```python
from build123d import *

# Parameters (mm, degrees)
EXTRU_MINCE1_DEPTH      = 8
ESQUISSE2_R             = 1.6
ENL_V_MAT_EXTRU_1_DEPTH = 109.260681026
ESQUISSE3_R             = 2
ENL_V_MAT_EXTRU_2_DEPTH = 5.5
ESQUISSE4_R             = 1.6
ENL_V_MAT_EXTRU_3_DEPTH = 109.260681026
ESQUISSE5_R             = 2
ENL_V_MAT_EXTRU_4_DEPTH = 5.5
ESQUISSE7_R             = 1.6
ENL_V_MAT_EXTRU_5_DEPTH = 102.558480966
ESQUISSE8_R             = 2
ENL_V_MAT_EXTRU_6_DEPTH = 5.5
CONG_1_R                = 2


with BuildPart() as part:
    # Esquisse1 → Extru.-Mince1 (new body)
    with BuildSketch(Plane(origin=(0, 0, 0), x_dir=(1, 0, 0), z_dir=(0, 1, 0))):
        with BuildLine():
            Line((0, 0), (19.803847577, 0))
            ThreePointArc((19.803847577, 0), (24.303847577, -1.205771366), (27.598076211, -4.5))
            Line((27.598076211, -4.5), (59.352341017, -59.5))
            ThreePointArc((59.352341017, -59.5), (62.646569651, -62.794228634), (67.146569651, -64))
            Line((67.146569651, -64), (86.950417228, -64))
            Line((86.950417228, -64), (86.950417228, -56))
            Line((86.950417228, -56), (67.146569651, -56))
            ThreePointArc((67.146569651, -56), (66.646569651, -55.866025404), (66.280544247, -55.5))
            Line((66.280544247, -55.5), (34.526279442, -0.5))
            ThreePointArc((34.526279442, -0.5), (28.303847577, 5.722431864), (19.803847577, 8))
            Line((19.803847577, 8), (0, 8))
            Line((0, 8), (0, 0))
        make_face()
    extrude(amount=EXTRU_MINCE1_DEPTH)

    # Esquisse2 → Enlèv. mat.-Extru.1 (cut, through all)
    with BuildSketch(Plane(origin=(0, 8, 0), x_dir=(1, 0, 0), z_dir=(0, 1, 0))):
        with Locations(Location((74.950417228, -60, 0), (0, 0, 270))):
            Circle(ESQUISSE2_R)
        with Locations(Location((12, 4, 0), (0, 0, 270))):
            Circle(ESQUISSE2_R)
    extrude(amount=-ENL_V_MAT_EXTRU_1_DEPTH, mode=Mode.SUBTRACT)

    # Esquisse3 → Enlèv. mat.-Extru.2 (cut)
    with BuildSketch(Plane.XZ):
        with Locations(Location((74.950417228, 60, 0), (0, 0, 270))):
            Circle(ESQUISSE3_R)
        with Locations(Location((12, -4, 0), (0, 0, 270))):
            Circle(ESQUISSE3_R)
    extrude(amount=-ENL_V_MAT_EXTRU_2_DEPTH, mode=Mode.SUBTRACT)

    # Esquisse4 → Enlèv. mat.-Extru.3 (cut, through all)
    with BuildSketch(Plane(origin=(0, 0, 0), x_dir=(-1, 0, 0), z_dir=(0, 0, -1))):
        with Locations((-5, 4)):
            Circle(ESQUISSE4_R)
    extrude(amount=ENL_V_MAT_EXTRU_3_DEPTH, mode=Mode.SUBTRACT)

    # Esquisse5 → Enlèv. mat.-Extru.4 (cut)
    with BuildSketch(Plane.XY.offset(-8)):
        with Locations((5, 4)):
            Circle(ESQUISSE5_R)
    extrude(amount=ENL_V_MAT_EXTRU_4_DEPTH, mode=Mode.SUBTRACT)

    # Esquisse7 → Enlèv. mat.-Extru.5 (cut, through all)
    with BuildSketch(Plane(origin=(18.75, 0, -10.825317547), x_dir=(0.499999999999998, 0, 0.8660254037844398), z_dir=(-0.8660254037844399, 0, 0.49999999999999806))):
        with Locations((49.450417228, 4)):
            Circle(ESQUISSE7_R)
    extrude(amount=-ENL_V_MAT_EXTRU_5_DEPTH, mode=Mode.SUBTRACT)

    # Esquisse8 → Enlèv. mat.-Extru.6 (cut)
    with BuildSketch(Plane(origin=(25.67820323, 0, -14.825317547), x_dir=(-0.49999999999999806, 0, -0.8660254037844398), z_dir=(0.8660254037844397, 0, -0.499999999999998))):
        with Locations((-49.450417228, 4)):
            Circle(ESQUISSE8_R)
    extrude(amount=-ENL_V_MAT_EXTRU_6_DEPTH, mode=Mode.SUBTRACT)

    # Congé1
    cong_1_edges = [part.edges().sort_by_distance(p)[0] for p in [
        (0, 0, -4),
        (9.901923789, 0, -8),
        (28.303847577, 0, -5.722431864),
        (50.403411844, 0, 28),
        (66.646569651, 0, 55.866025404),
        (77.048493439, 0, 56),
        (86.950417228, 0, 60),
        (0, 4, -8),
        (86.950417228, 4, 56),
    ]]
    fillet(cong_1_edges, radius=CONG_1_R - 0.0001)  # a hair under: the kernel refuses the full size


solid = part.part
```
Geometry check sheet. Reference: the model listing, model coordinates, mm. A direction names the side the tool comes from. Give positions to 0.01 mm unless a question says otherwise; leave off trailing zeros. Write each loop counter-clockwise with the first axis right and the second up, starting at its lowest first coordinate (ties: lowest second). Pieces come first, ordered by that corner, then holes.
1) Gauge pin test, flat ends, axial feed: pin 1 (1.8 mm diameter, centred on x = 79.5, y = 5.5, fed in from -Z); pin 2 (2 mm diameter, centred on y = 1.5, z = 19, fed in from -X); pin 3 (2.5 mm diameter, centred on x = 9.5, y = 3, fed in from +Z). Record the tip position at first contact, or that the pin passes through.
2) Material ranges on L1, parallel to Y at x = 5, z = -5.7; L2, parallel to Z at x = 8.5, y = 3.5; L3, parallel to X at y = 4, z = -1.05, recorded low to high.
3) Section check B-B, the plane y = 4. State how many separate pieces and enclosed holes the cut face has, and give its area (3 significant figures).
4) Release check for a two-part mould opening along Z. For faces 1 (the flat face through (10, 4, 0)), 2 (the cylindrical face through (14, 3, -4)), 3 (the flat face through (0, 5, -3)) record: pulls with the +Z half, pulls with the -Z half, needs draft (parallel to the pull), parting line crosses it, or undercut.
5) Section check C-C, the plane x = 79.5. Record the boundary of the cut face in (y, z), and give its area (3 significant figures).
6) Access from +Z, -Z, +X, -X, +Y, -Y to the whole of each face (thin tool, end or side, straight path). Record for faces 4 (the cylindrical face through (86.35, 0.57, 60.96)), 5 (the flat face through (76, 5, 56)).
Computed:
1. pin 1: stops at z = 56
1. pin 2: stops at x = 35.39
1. pin 3: stops at z = 0
2. L1: y = 0 to 2, 6 to 8
2. L2: z = -8 to 0
2. L3: x = 0 to 3.4, 6.6 to 33.52
3. separate pieces: 3
3. enclosed holes: 2
3. area: 889 mm2
4. face 1: pulls with the +Z half
4. face 2: undercut
4. face 3: needs draft
5. outline: (0, 58) arc R2 ccw to (2, 56) - (8, 56) - (8, 64) - (0, 64) - close
5. area: 63.1 mm2
6. face 4: +Z, -Z, +X, -Y
6. face 5: -Z, +X, +Y, -Y
